The listing builds one solid part. Answer for the finished solid, in the listing's coordinates (mm). Give positions to 0.01 mm unless a question says otherwise; leave off trailing zeros. Order: outer loops, then holes, each group sorted by start corner. A loop starts at its lowest first (then second) coordinate and runs counter-clockwise, first axis right, second up.
```python
from build123d import *

# Parameters (mm, degrees)
SKETCH1_W           = 355.6
SKETCH1_H           = 50.8
BOSS_EXTRUDE1_DEPTH = 4.7625
BOSS_EXTRUDE2_DEPTH = 4.7625
SKETCH3_W           = 6.858
SKETCH3_H           = 19.471321321
SKETCH3_W_2         = 6.35
SKETCH3_H_2         = 18.963321321
CUT_EXTRUDE1_DEPTH  = 198.660000053
SKETCH4_W           = 1.5875
SKETCH4_H           = 15.621
SKETCH4_H_2         = 22.553060346
CUT_EXTRUDE2_DEPTH  = 198.660000053
CUT_EXTRUDE3_START  = -4.7625
CUT_EXTRUDE3_DEPTH  = 4.7625
SKETCH6_W           = 0.3175
SKETCH6_H           = 19.471321321
CUT_EXTRUDE4_DEPTH  = 197.233230563
SKETCH7_W           = 155.575
SKETCH7_H           = 76.528060346
CUT_EXTRUDE5_DEPTH  = 197.233230563


# Read off the part's stored shape, not the designer's step: Cut-Extrude3
with BuildPart() as part:
    # Sketch1 → Boss-Extrude1 (new body)
    with BuildSketch(Plane(origin=(0, 0, 0), x_dir=(1, 0, 0), z_dir=(0, 1, 0))):
        Rectangle(SKETCH1_W, SKETCH1_H)
    extrude(amount=BOSS_EXTRUDE1_DEPTH)

    # Sketch2 → Boss-Extrude2 (add)
    with BuildSketch(Plane(origin=(0, 4.7625, 0), x_dir=(1, 0, 0), z_dir=(0, 1, 0))):
        Polygon((177.8, -25.4), (88.9, -86.220381667), (76.2, -86.220381667), (76.2, -25.4), align=None)
        Polygon((-177.8, -25.4), (-88.9, -86.220381667), (-76.2, -86.220381667), (-76.2, -25.4), align=None)
    extrude(amount=-BOSS_EXTRUDE2_DEPTH)

    # Sketch3 → Cut-Extrude1 (cut, through all)
    # profile 1 of 6: a face of its own
    with BuildSketch(Plane(origin=(0, 4.7625, 0), x_dir=(1, 0, 0), z_dir=(0, 1, 0))):
        with Locations((-174.625, 0.043339339)):
            Rectangle(SKETCH3_W, SKETCH3_H)
        with Locations((-174.625, 0.04333934)):
            Rectangle(SKETCH3_W_2, SKETCH3_H_2, mode=Mode.SUBTRACT)
    # profile 2 of 6: a face of its own
    with BuildSketch(Plane(origin=(0, 4.7625, 0), x_dir=(1, 0, 0), z_dir=(0, 1, 0))):
        with Locations((-79.375, -53.931660661)):
            Rectangle(SKETCH3_W, SKETCH3_H)
        with Locations((-79.375, -53.931660661)):
            Rectangle(SKETCH3_W_2, SKETCH3_H_2, mode=Mode.SUBTRACT)
    # profile 3 of 6: a face of its own
    with BuildSketch(Plane(origin=(0, 4.7625, 0), x_dir=(1, 0, 0), z_dir=(0, 1, 0))):
        with Locations((-79.375, 0.043339339)):
            Rectangle(SKETCH3_W, SKETCH3_H)
        with Locations((-79.375, 0.04333934)):
            Rectangle(SKETCH3_W_2, SKETCH3_H_2, mode=Mode.SUBTRACT)
    # profile 4 of 6: a face of its own
    with BuildSketch(Plane(origin=(0, 4.7625, 0), x_dir=(1, 0, 0), z_dir=(0, 1, 0))):
        with Locations((79.375, 0.043339339)):
            Rectangle(SKETCH3_W, SKETCH3_H)
        with Locations((79.375, 0.04333934)):
            Rectangle(SKETCH3_W_2, SKETCH3_H_2, mode=Mode.SUBTRACT)
    # profile 5 of 6: a face of its own
    with BuildSketch(Plane(origin=(0, 4.7625, 0), x_dir=(1, 0, 0), z_dir=(0, 1, 0))):
        with Locations((79.375, -53.931660661)):
            Rectangle(SKETCH3_W, SKETCH3_H)
        with Locations((79.375, -53.931660661)):
            Rectangle(SKETCH3_W_2, SKETCH3_H_2, mode=Mode.SUBTRACT)
    # profile 6 of 6: a face of its own
    with BuildSketch(Plane(origin=(0, 4.7625, 0), x_dir=(1, 0, 0), z_dir=(0, 1, 0))):
        with Locations((174.625, 0.043339339)):
            Rectangle(SKETCH3_W, SKETCH3_H)
        with Locations((174.625, 0.04333934)):
            Rectangle(SKETCH3_W_2, SKETCH3_H_2, mode=Mode.SUBTRACT)
    extrude(amount=-CUT_EXTRUDE1_DEPTH, mode=Mode.SUBTRACT)


with BuildPart() as body_2:
    # of the pieces the cut leaves, the one that is kept (cut_extrude1_keep)
    add(part.part.solids().sort_by_distance((-177.8, 0, -25.4))[0])

    # Sketch4 → Cut-Extrude2 (cut, through all)
    with BuildSketch(Plane(origin=(0, 4.7625, 0), x_dir=(1, 0, 0), z_dir=(0, 1, 0))):
        Polygon((-176.2125, -26.486078244), (-176.2125, -9.692321321), (-177.8, -9.692321321), (-177.8, -25.4), align=None)
        with Locations((-177.00625, 17.5895)):
            Rectangle(SKETCH4_W, SKETCH4_H)
        with Locations((-76.99375, -74.943851494)):
            Rectangle(SKETCH4_W, SKETCH4_H_2)
        with Locations((76.99375, -74.943851494)):
            Rectangle(SKETCH4_W, SKETCH4_H_2)
        Polygon((177.8, -9.692321321), (176.2125, -9.692321321), (176.2125, -26.486078244), (177.8, -25.4), align=None)
        with Locations((177.00625, 17.5895)):
            Rectangle(SKETCH4_W, SKETCH4_H)
    extrude(amount=-CUT_EXTRUDE2_DEPTH, mode=Mode.SUBTRACT)

    # Cut-Extrude3 outline → Cut-Extrude3 (cut)
    with BuildSketch(Plane(origin=(0, 4.7625, 0), x_dir=(1, 0, 0), z_dir=(0, 1, 0)).offset(CUT_EXTRUDE3_START)):
        with BuildLine():
            Line((-76.2, -9.692321321), (-76.2, -25.4))
            Line((-76.2, -25.4), (76.2, -25.4))
            Line((76.2, -25.4), (76.2, -9.692321321))
            Line((76.2, -9.692321321), (75.946, -9.692321321))
            Line((75.946, -9.692321321), (75.946, 9.779))
            ThreePointArc((75.946, 9.779), (70.210694069, 11.958939555), (64.119988035, 12.7))
            Line((64.119988035, 12.7), (-64.119988035, 12.7))
            ThreePointArc((-64.119988035, 12.7), (-70.210694069, 11.958939555), (-75.946, 9.779))
            Line((-75.946, 9.779), (-75.946, -9.692321321))
            Line((-75.946, -9.692321321), (-76.2, -9.692321321))
        make_face()
    extrude(amount=CUT_EXTRUDE3_DEPTH, mode=Mode.SUBTRACT)

    # Sketch6 → Cut-Extrude4 (cut, through all)
    with BuildSketch(Plane(origin=(0, 4.7625, 0), x_dir=(1, 0, 0), z_dir=(0, 1, 0))):
        with Locations((-82.96275, 0.043339339)):
            Rectangle(SKETCH6_W, SKETCH6_H)
        with Locations((-82.96275, -53.931660661)):
            Rectangle(SKETCH6_W, SKETCH6_H)
        with Locations((82.96275, -53.931660661)):
            Rectangle(SKETCH6_W, SKETCH6_H)
        with Locations((82.96275, 0.043339339)):
            Rectangle(SKETCH6_W, SKETCH6_H)
    extrude(amount=-CUT_EXTRUDE4_DEPTH, mode=Mode.SUBTRACT)

    # Sketch7 → Cut-Extrude5 (cut, through all)
    with BuildSketch(Plane(origin=(0, 4.7625, 0), x_dir=(1, 0, 0), z_dir=(0, 1, 0))):
        with Locations((0, -47.956351494)):
            Rectangle(SKETCH7_W, SKETCH7_H)
    extrude(amount=-CUT_EXTRUDE5_DEPTH, mode=Mode.SUBTRACT)


solid = body_2.part
```
1) Find section A-A (z = 21.5). Write down the section's boundary in (x, y), then the cut area to 4 significant figures.
Geometry says:
outline: (-176.21, 0) - (-77.79, 0) - (-77.79, 4.76) - (-176.21, 4.76) - close; (77.79, 0) - (176.21, 0) - (176.21, 4.76) - (77.79, 4.76) - close
area: 937.5 mm2
2) Find section D-D (x = 59). Write down the section's boundary in (y, z).
Geometry says:
outline: (0, -25.4) - (4.76, -25.4) - (4.76, -12.7) - (0, -12.7) - close
3) Find section B-B (z = -6.5). Write down the section's boundary in (x, y).
Geometry says:
outline: (-171.2, 0) - (-83.12, 0) - (-83.12, 4.76) - (-171.2, 4.76) - close; (83.12, 0) - (171.2, 0) - (171.2, 4.76) - (83.12, 4.76) - close
4) Given P1, Ø1, axis at x = -122.5, y = 4, coming from the +Z side; P2, Ø2.5, axis at y = 1.5, z = 77.5, coming from the +X side; P3, Ø1, axis at x = 72.5, z = -14, coming from the -Y side; P4, Ø1.4, axis at y = 2, z = 0, coming from the +X side, each flat-ended and moving along its own axis, determine where each tip first touches the part or whether it passes through.
Geometry says:
P1: stops at z = 63.58
P2: stops at x = 103.47
P3: stops at y = 0
P4: stops at x = 171.2
5) Straight lines are drawn through the part: probe 1 along Z at (x, y) = (80, 1.6); probe 2 along X at (y, z) = (4.5, 11); probe 3 along Z at (x, y) = (63, 2.4). For each, find the intervals that lie inside material, in ascending order.
Geometry says:
probe 1: z = -25.4 to -9.78, 9.69 to 44.2, 63.67 to 86.22
probe 2: x = -176.21 to -77.79, 77.79 to 176.21
probe 3: z = -25.4 to -12.7
